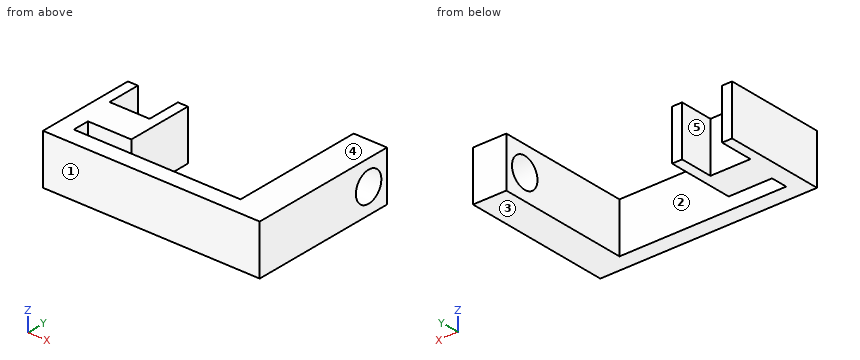
from build123d import *

# Parameters (mm, degrees)
EXTRUDE_1_DEPTH     = 15
SKETCH_5_R          = 4.5
CUT_EXTRUDE_1_DEPTH = 15


with BuildPart() as part:
    # Эскиз4 → Бобышка-Вытянуть1 (new body)
    with BuildSketch(Plane.XY):
        Polygon((0, 0), (0, -20), (0, -30), (65, -30), (65, 15), (55, 15), (55, -25), (5, -25), (5, -20), (18, -20), (18, 0), (15, 0), (15, -10), (3, -10), (3, 0), align=None)
    extrude(amount=EXTRUDE_1_DEPTH)

    # Эскиз5 → Вырез-Вытянуть1 (cut)
    with BuildSketch(Plane(origin=(65, 0, 0), x_dir=(0, 0, -1), z_dir=(1, 0, 0))):
        with Locations((-7.5, 8.5)):
            Circle(SKETCH_5_R)
    extrude(amount=-CUT_EXTRUDE_1_DEPTH, mode=Mode.SUBTRACT)


solid = part.part
Input: part model. Units: mm. Frame: model coordinates. Face numbers are marked on the shaded views. A direction names the side the tool comes from. Round coordinates to 2 decimals unless told otherwise and drop trailing zeros. Loops run counter-clockwise (first coordinate to the right, second up) from the corner with the lowest first, then second, coordinate; pieces in that order, holes last. Notation, with made-up numbers: (30, 24) -> (66, 24) arc R24 ccw to (66, 49) -> close; hole circle Ø10 at (74, -1). An arc over 180 degrees is marked (long way). Answer as a JSON object with one key per item and string values. Group by question number.
1) Reachability of the marked faces 4 and 5 from +Z, -Z, +X, -X, +Y, -Y: full face, straight path, thin tool, end or side. Return the list, or none.
2) Section query D-D on x = 61. Output: boundary loops of the cut face in (y, z), plus the area to 3 significant figures.
3) Section query B-B on z = 7.5. Output: boundary loops of the cut face in (x, y).
4) Ray query, L1, parallel to X at y = -6.5, z = 13.5; L2, parallel to Y at x = 57.75, z = 7.5; L3, parallel to X at y = -22, z = 10.75. Return the intervals inside material, ascending.
5) Section query C-C on y = -4. Output: boundary loops of the cut face in (x, z).
6) Pin query (flat end, axial travel): pin 1 (4.5 mm diameter, centred on x = 26, z = 7, fed in from +Y); pin 2 (2 mm diameter, centred on x = 14.5, z = 10, fed in from +Y); pin 3 (3.5 mm diameter, centred on x = 10.5, z = 10, fed in from +Y). Return the tip coordinate at first contact, or that it passes through.
7) Section query A-A on y = 8.5. Output: boundary loops of the cut face in (x, z), plus the area to 3 significant figures.
8) Draft query along Y for the marked faces 1, 2 and 3. Return one class per face: +Y half, -Y half, draft (parallel to the pull), parting line (faces both ways), or undercut.
Reply:
{
 "1": {"face 4": "+Z, +X, -X, +Y, -Y", "face 5": "+Z, -Z, +Y"},
 "2": {"outline": "(-30, 0) -> (15, 0) -> (15, 15) -> (-30, 15) -> close; hole circle Ø9 at (8.5, 7.5)", "area": "611 mm2"},
 "3": {"outline": "(0, -30) -> (65, -30) -> (65, 4) -> (55, 4) -> (55, -25) -> (5, -25) -> (5, -20) -> (18, -20) -> (18, 0) -> (15, 0) -> (15, -10) -> (3, -10) -> (3, 0) -> (0, 0) -> close; (55, 13) -> (65, 13) -> (65, 15) -> (55, 15) -> close"},
 "4": {"L1": "x = 0 to 3, 15 to 18, 55 to 65", "L2": "y = -30 to 4, 13 to 15", "L3": "x = 0 to 5, 55 to 65"},
 "5": {"outline": "(0, 0) -> (3, 0) -> (3, 15) -> (0, 15) -> close; (15, 0) -> (18, 0) -> (18, 15) -> (15, 15) -> close; (55, 0) -> (65, 0) -> (65, 15) -> (55, 15) -> close"},
 "6": {"pin 1": "stops at y = -25", "pin 2": "stops at y = 0", "pin 3": "stops at y = -10"},
 "7": {"outline": "(55, 0) -> (65, 0) -> (65, 3) -> (55, 3) -> close; (55, 12) -> (65, 12) -> (65, 15) -> (55, 15) -> close", "area": "60.0 mm2"},
 "8": {"face 1": "-Y half", "face 2": "undercut", "face 3": "draft"}
}
